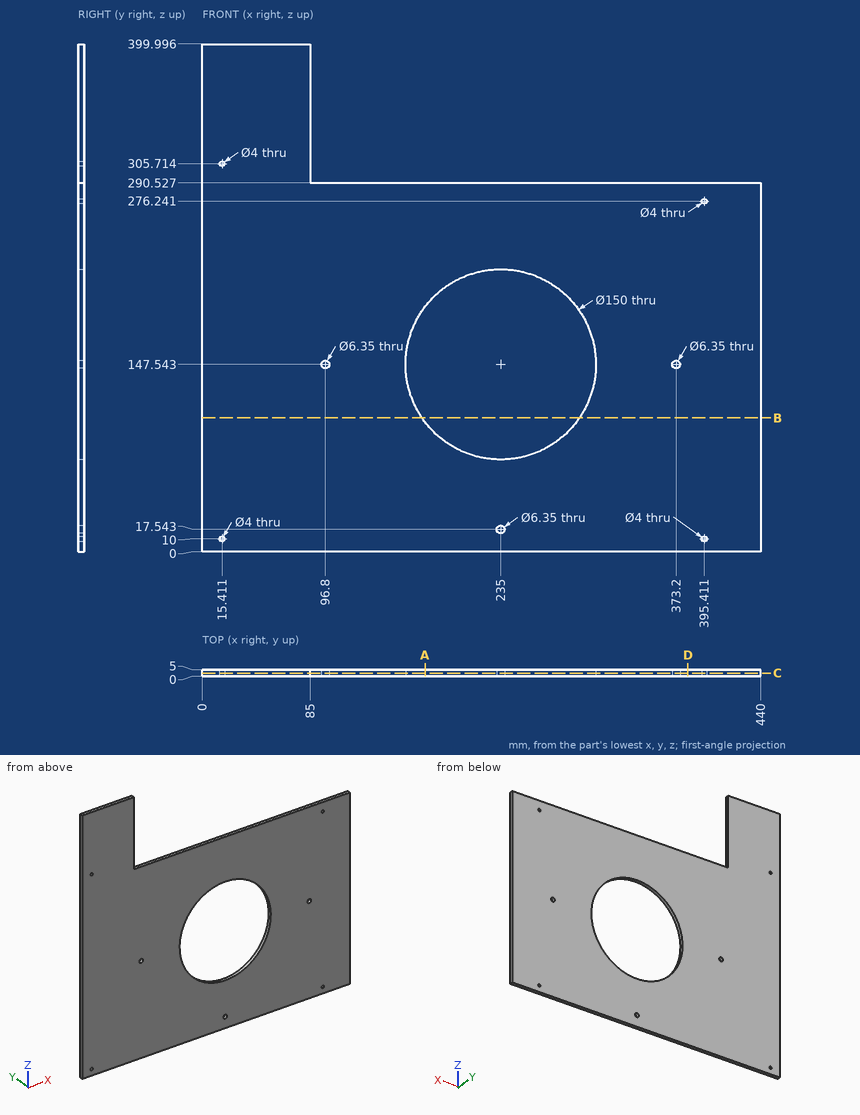
Geometry check sheet. Reference: drawing and pictorial views, mm from the part's lowest x, y, z. Coordinates: 2 decimals unless noted, no trailing zeros. Write each loop counter-clockwise with the first axis right and the second up, starting at its lowest first coordinate (ties: lowest second). Pieces come first, ordered by that corner, then holes. Notation, with made-up numbers: M 2,62 L 11,62 A32 cw 11,93 Z; hole C 25,49.5 d5. An arc over 180 degrees is marked long. Write item = value, one per line. Start each with the question number.
1. Sectioned sample at B-B (z = 105.5). Record the cut outline in (x, y), then the cut area to 3 significant figures.
2. Thickness scan on probe 1 along X at (y, z) = (3.9, 348); probe 2 along Z at (x, y) = (221, 1) (1 decimal); probe 3 along X at (y, z) = (3, 149.5) (1 decimal). Record the ranges inside material, lowest first.
3. Sectioned sample at C-C (y = 2.25). State how many separate pieces and enclosed holes the cut face has, then the cut area to 3 significant figures.
4. Sectioned sample at A-A (x = 175.5). Record the cut outline in (y, z), then the cut area to 3 significant figures.
5. Sectioned sample at D-D (x = 382.5). Record the cut outline in (y, z).
6. Go/stop test with flat-tipped pins: pin 1 (5 mm diameter, centred on x = 15.41, z = 10, fed in from -Y); pin 2 (1.5 mm diameter, centred on x = 144, y = 3.5, fed in from +Z). Record where each tip stops, or that it passes through.
The answers:
q1.outline = M 0,0 L 172.89,0 L 172.89,5 L 0,5 Z; M 297.11,0 L 440,0 L 440,5 L 297.11,5 Z
q1.area = 1,580 mm²
q2.probe_1 = 0 to 85
q2.probe_2 = 0 to 73.9, 221.2 to 290.5
q2.probe_3 = 0 to 94.3, 99.3 to 160, 310 to 370.7, 375.7 to 440
q3.separate_pieces = 1
q3.enclosed_holes = 8
q3.area = 119,000 mm²
q4.outline = M 0,0 L 5,0 L 5,101.88 L 0,101.88 Z; M 0,193.2 L 5,193.2 L 5,290.53 L 0,290.53 Z
q4.area = 996 mm²
q5.outline = M 0,0 L 5,0 L 5,290.53 L 0,290.53 Z
q6.pin_1 = 0
q6.pin_2 = 290.53
